Part model, mm, in its own coordinate system. Face numbers are marked on the shaded views. A direction names the side the tool comes from. Give positions to 0.01 mm unless a question says otherwise; leave off trailing zeros. Write each loop counter-clockwise with the first axis right and the second up, starting at its lowest first coordinate (ties: lowest second). Pieces come first, ordered by that corner, then holes. Notation, with made-up numbers: M -22,16 L -18,16 A17 ccw -18,29 Z; hole C -39,-31.75 d5. An arc over 180 degrees is marked long. Answer as CSV lines item,"result". Start each with the question number.
Item 1: Band-saw the part on C-C, the plane z = 7.5. List the corners of the cut face in (x, y), then the cut area to 3 significant figures.
Item 2: Band-saw the part on B-B, the plane y = 2.45. List the corners of the cut face in (x, z).
Item 3: Band-saw the part on A-A, the plane z = 4.5. List the corners of the cut face in (x, y), then the cut area to 3 significant figures.
Item 4: 3-axis set-ups, long thin cutter, end or side, ignore diameter. For the marked faces 1 and 2: which of +Z, -Z, +X, -X, +Y, -Y reach the whole face in a straight line?
Item 5: Wall check: L1, parallel to Z at x = 2.5, y = 2.6; L2, parallel to X at y = 2.1, z = 4.5; L3, parallel to X at y = 2.1, z = 6.5. Give the ranges that are in metal, low to high. Write a range as from..to.
Item 6: Band-saw the part on D-D, the plane x = -8. List the corners of the cut face in (y, z).
from build123d import *

# Parameters (mm, degrees)
SKETCH1_W               = 20
SKETCH1_H               = 20
BOSS_EXTRUDE1_DEPTH     = 3
CUT_EXTRUDE1_DEPTH      = 1
CUT_EXTRUDE1_DEPTH_BACK = 4


with BuildPart() as part:
    # Sketch1 → Boss-Extrude1 (new body)
    with BuildSketch(Plane(origin=(0, 0, 0), x_dir=(1, 0, 0), z_dir=(0, 1, 0))):
        Rectangle(SKETCH1_W, SKETCH1_H)
    extrude(amount=BOSS_EXTRUDE1_DEPTH)

    # Sketch2 → Cut-Extrude1 (cut, two sides)
    with BuildSketch(Plane(origin=(0, 3, 0), x_dir=(1, 0, 0), z_dir=(0, 1, 0))) as cut_extrude1_sk:
        Polygon((-5, -10), (-10, 0), (-10, -10), align=None)
        Polygon((0, 0), (-5, -10), (5, -10), align=None)
        Polygon((10, 0), (5, -10), (10, -10), align=None)
    extrude(amount=CUT_EXTRUDE1_DEPTH, mode=Mode.SUBTRACT)
    extrude(cut_extrude1_sk.sketch, amount=-CUT_EXTRUDE1_DEPTH_BACK, mode=Mode.SUBTRACT)


solid = part.part
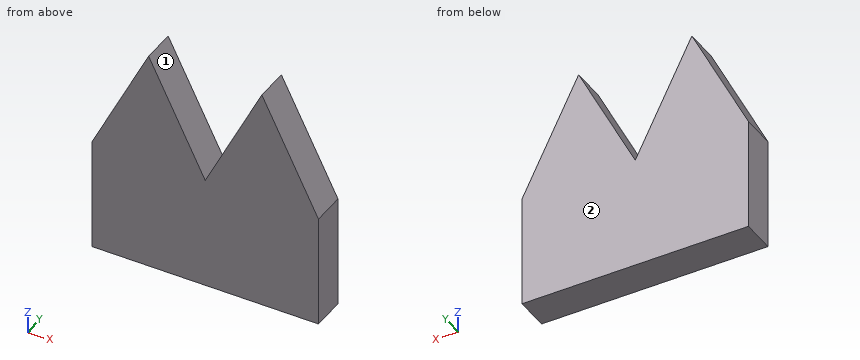
Output:
1,outline,"M -6.25,0 L -3.75,0 L -3.75,3 L -6.25,3 Z; M 3.75,0 L 6.25,0 L 6.25,3 L 3.75,3 Z"
1,area,"15.0 mm²"
2,outline,"M -10,-10 L 10,-10 L 10,0 L 5,10 L 0,0 L -5,10 L -10,0 Z"
3,outline,"M -7.75,0 L -2.25,0 L -2.25,3 L -7.75,3 Z; M 2.25,0 L 7.75,0 L 7.75,3 L 2.25,3 Z"
3,area,"33.0 mm²"
4,face 1,"+Z, +Y, -Y"
4,face 2,"+Z, -Z, +X, -X, +Y"
5,L1,"-10..5"
5,L2,"-7.75..-2.25, 2.25..7.75"
5,L3,"-6.75..-3.25, 3.25..6.75"
6,outline,"M 0,-10 L 3,-10 L 3,4 L 0,4 Z"
